Design review of the part built by this model. Coordinates are the model's own, in mm. Round coordinates to 2 decimals unless told otherwise and drop trailing zeros. Loops run counter-clockwise (first coordinate to the right, second up) from the corner with the lowest first, then second, coordinate; pieces in that order, holes last. Notation, with made-up numbers: M -7.5,-40 L 50.5,-40 A12 cw 50.5,-36 Z; hole C 10.5,-26.5 d4. An arc over 180 degrees is marked long. One line per item, written item: value. Start each with the question number.
Item 1: For line 1 along Y through (x, z) = (-218.95, 2); line 2 along Z through (x, y) = (-217, 87); line 3 along X through (y, z) = (90, 7.75), list the stretches that pass through material, from the lowest coordinate up.
Item 2: We need section A-A (z = 4). Write out the cut boundary in (x, y), then the cut area to 3 significant figures.
Item 3: Clearance check with flat-ended pins moving along their axes: pin 1 (2 mm diameter, centred on y = 92.5, z = 6.5, fed in from +X); pin 2 (2 mm diameter, centred on y = 88.5, z = 7, fed in from -X); pin 3 (1.5 mm diameter, centred on x = -218, y = 83.5, fed in from -Z); pin 4 (1.5 mm diameter, centred on x = -219, y = 88, fed in from -Z). State where each tip first meets the part, or that it passes through.
Item 4: We need section B-B (x = -217.85). Write out the cut boundary in (y, z).
Item 5: Mouldability with a two-part tool opening along Z and no side actions: class faces 1 (the flat face through (-215.68, 90.81, 7.97)), 2 (the flat face through (-217.063, 88.031, 5.944)), 3 (the flat face through (-217.87, 85.38, 2.88)) as released by +Z, released by -Z, zero draft, split by the parting line, or undercut.
Item 6: We need section D-D (z = 5.5). Write out the cut boundary in (x, y).
Item 7: We need section C-C (y = 84.25). Write out the cut boundary in (x, z), then the cut area to 3 significant figures.
from build123d import *

# Parameters (mm, degrees)
BOX216_W                  = 0.5
BOX216_H                  = 1
BOX216_DEPTH              = 11
BOX217_W                  = 0.5
BOX217_H                  = 1
BOX217_DEPTH              = 16
BOX217_ROLL_ANGLE         = 49
BOX218_W                  = 0.5
BOX218_H                  = 1
BOX218_DEPTH              = 16
BOX218_ROLL_ANGLE         = -49
BOX215_W                  = 0.5
BOX215_H                  = 1
BOX215_DEPTH              = 11
FUSION016_PLACEMENT_ANGLE = -22


with BuildPart() as cubo216:
    # Box216 → Box216 (new body)
    with BuildSketch(Plane(origin=(0, 12, 0.5), x_dir=(1, 0, 0), z_dir=(0, 0, 1))):
        with Locations((0.25, 0.5)):
            Rectangle(BOX216_W, BOX216_H)
    extrude(amount=BOX216_DEPTH)


with BuildPart() as cubo217:
    # Box217 → Box217 (new body)
    with BuildSketch(Plane.XY):
        with Locations((0.25, 0.5)):
            Rectangle(BOX217_W, BOX217_H)
    extrude(amount=BOX217_DEPTH)


with BuildPart() as cubo217_1:
    # Box217 roll: moved
    add(cubo217.part.rotate(Axis((0, 0, 0), (1, 0, 0)), BOX217_ROLL_ANGLE))


with BuildPart() as cubo217_2:
    # Box217 placement: moved
    add(cubo217_1.part.moved(Location((0, 12, 0.5))))


with BuildPart() as cubo218:
    # Box218 → Box218 (new body)
    with BuildSketch(Plane.XY):
        with Locations((0.25, 0.5)):
            Rectangle(BOX218_W, BOX218_H)
    extrude(amount=BOX218_DEPTH)


with BuildPart() as cubo218_1:
    # Box218 roll: moved
    add(cubo218.part.rotate(Axis((0, 0, 0), (1, 0, 0)), BOX218_ROLL_ANGLE))


with BuildPart() as cubo218_2:
    # Box218 placement: moved
    add(cubo218_1.part.moved(Location((0, 0.4, 1.3))))


with BuildPart() as fusion016:
    # Box215 → Box215 (new body)
    with BuildSketch(Plane.XY.offset(0.5)):
        with Locations((0.25, 0.5)):
            Rectangle(BOX215_W, BOX215_H)
    extrude(amount=BOX215_DEPTH)

    # Fusion016: union Cubo216, Cubo217, Cubo218
    add(cubo216.part)
    add(cubo217_2.part)
    add(cubo218_2.part)


with BuildPart() as fusion016_1:
    # Fusion016 placement: moved
    add(fusion016.part.moved(Location((-219.5, 82, 0))).rotate(Axis((-219.5, 82, 0), (0, 0, 1)), FUSION016_PLACEMENT_ANGLE))


solid = fusion016_1.part
A:
1. line 1: 82.03 to 82.86, 83.08 to 83.36
1. line 2: 4.47 to 5.8, 6.09 to 7.41
1. line 3: -216.27 to -215.73
2. outline: M -219.5,82 L -219.04,81.81 L -218.66,82.74 L -219.13,82.93 Z; M -218.19,85.25 L -217.72,85.06 L -217.15,86.48 L -217.62,86.66 Z; M -216.51,89.39 L -216.05,89.21 L -215.48,90.62 L -215.94,90.81 Z; M -215,93.13 L -214.54,92.94 L -214.17,93.87 L -214.63,94.05 Z
2. area: 2.52 mm2
3. pin 1: x = -214.31
3. pin 2: x = -217.28
3. pin 3: z = 0.74
3. pin 4: through
4. outline: M 84.75,2.38 L 86.08,3.46 L 86.08,4.78 L 84.75,3.71 Z; M 84.75,8.18 L 86.08,7.1 L 86.08,8.43 L 84.75,9.5 Z
5. face 1: undercut
5. face 2: zero draft
5. face 3: released by -Z
6. outline: M -219.5,82 L -219.04,81.81 L -218.66,82.74 L -219.13,82.93 Z; M -217.54,86.85 L -217.08,86.66 L -216.12,89.02 L -216.59,89.21 Z; M -215,93.13 L -214.54,92.94 L -214.17,93.87 L -214.63,94.05 Z
7. outline: M -218.59,1.74 L -218.05,1.91 L -218.05,3.24 L -218.59,3.06 Z; M -218.59,8.82 L -218.05,8.65 L -218.05,9.97 L -218.59,10.15 Z
7. area: 1.43 mm2
